For this review, take the finished solid that the model builds, in its own axes (mm). Face numbers are marked on the shaded views. A direction names the side the tool comes from. Coordinates: 2 decimals unless noted, no trailing zeros. Write each loop counter-clockwise with the first axis right and the second up, starting at its lowest first coordinate (ties: lowest second). Pieces come first, ordered by that corner, then holes.
1) We need section D-D on z = -5. Write out the cut boundary in (x, y), then the cut area to 3 significant figures.
2) We need section A-A on x = 0. Write out the cut boundary in (y, z), then the cut area to 4 significant figures.
3) We need section B-B on z = 73.5. Give the number of separate pieces and of enclosed holes in the cut face, then the cut area to 3 significant figures.
4) For the marked faces 5, 6 and 7, list the 3-axis set-ups (+Z, -Z, +X, -X, +Y, -Y) from which the entire face can be reached by the end or side of a thin tool; tool diameter is ignored.
5) To check wall thickness, follow line 1 along Z through (x, y) = (0, 0.5); line 2 along X through (y, z) = (9.25, 73.5); line 3 along X through (y, z) = (7, 21.5). State the ranges of each line that lie inside material, in increasing order.
6) We need section C-C on x = 5.5. Write out the cut boundary in (y, z), then the cut area to 4 significant figures.
7) Insertion check: P1, Ø1.5, axis at x = -19.5, z = 22, coming from the +Y side; P2, Ø12, axis at x = 5, z = 68, coming from the +Y side; P3, Ø1.9, axis at x = 17.5, z = 65, coming from the +Y side; P4, Ø2.5, axis at x = -17, z = 29.5, coming from the -Y side. Each pin has a flat end and moves straight along its axis. Give the tip position at first contact, or say it passes through.
8) Mouldability with a two-part tool opening along X and no side actions: class the marked faces 1, 2, 3 and 4 as pulls with the +X half, pulls with the -X half, needs draft (parallel to the pull), parting line crosses it, or undercut.
from build123d import *

# Parameters (mm, degrees)
BOSS_EXTRUDE1_DEPTH = 95
CUT_EXTRUDE1_DEPTH  = 1
CUT_EXTRUDE2_DEPTH  = 1
CUT_EXTRUDE4_DEPTH  = 2
CUT_EXTRUDE5_DEPTH  = 2
FILLET1_R           = 2
FILLET2_R           = 5
FILLET3_R           = 5
SKETCH11_R          = 3.25
SKETCH11_R_2        = 1.9
BOSS_EXTRUDE2_DEPTH = 1.5
SKETCH13_R          = 2.5
BOSS_EXTRUDE3_DEPTH = 7.4
SKETCH14_R          = 1.9
BOSS_EXTRUDE4_DEPTH = 1
SKETCH15_R          = 1.65
CUT_EXTRUDE7_DEPTH  = 15
SKETCH16_R          = 2.75
CUT_EXTRUDE8_DEPTH  = 1
SKETCH17_R          = 1
CUT_EXTRUDE9_DEPTH  = 2
SKETCH18_W          = 37.144162516
SKETCH18_H          = 8.058946384
CUT_EXTRUDE10_DEPTH = 3
SKETCH19_R          = 1
SKETCH19_R_2        = 1.4
CUT_EXTRUDE11_DEPTH = 3
SKETCH20_W          = 42.739965368
SKETCH20_H          = 1.5
BOSS_EXTRUDE5_DEPTH = 10
FILLET4_R           = 10
SKETCH21_W          = 42.739965368
SKETCH21_H          = 1.5
BOSS_EXTRUDE6_DEPTH = 10
FILLET5_R           = 10
SKETCH22_R          = 2.5
CUT_EXTRUDE12_DEPTH = 10
SKETCH23_R          = 2.5
CUT_EXTRUDE13_DEPTH = 4.5


with BuildPart() as part:
    # Sketch1 → Boss-Extrude1 (new body)
    with BuildSketch(Plane.XY):
        Polygon((-26.114805518, 0), (-27.425, 25), (-24.921569135, 25), (-23.742394101, 2.5), (23.742394101, 2.5), (24.921569135, 25), (27.425, 25), (26.114805518, 0), align=None)
    extrude(amount=BOSS_EXTRUDE1_DEPTH)

    # Sketch2 → Cut-Extrude1 (cut)
    with BuildSketch(Plane(origin=(23.546701863, -1.234030354, 0), x_dir=(0, 0, 1), z_dir=(-0.9986295347545742, 0.052335956242940705, 0))):
        Polygon((93, 3.739154736), (93, 24.853460661), (2, 24.853460661), (2, 3.739154736), (0, 3.739154736), (0, 26.853460661), (95, 26.853460661), (95, 3.739154736), align=None)
    extrude(amount=-CUT_EXTRUDE1_DEPTH, mode=Mode.SUBTRACT)

    # Sketch4 → Cut-Extrude2 (cut)
    with BuildSketch(Plane(origin=(-23.546701863, -1.234030354, 0), x_dir=(0, 0, -1), z_dir=(0.9986295347545742, 0.052335956242940414, 0))):
        Polygon((-95, 3.739154736), (-93, 3.739154736), (-93, 24.754638821), (-2, 24.754638821), (-2, 3.739154736), (0, 3.739154736), (0, 26.754638821), (-95, 26.754638821), align=None)
    extrude(amount=-CUT_EXTRUDE2_DEPTH, mode=Mode.SUBTRACT)

    # Sketch9 → Cut-Extrude4 (cut)
    with BuildSketch(Plane.XY.offset(95)):
        Polygon((-24.741023636, 2.447664044), (-24.691358668, 1.5), (24.691358668, 1.5), (24.743766447, 2.5), (23.742394101, 2.5), (-23.742394101, 2.5), (-24.743766447, 2.5), align=None)
    extrude(amount=-CUT_EXTRUDE4_DEPTH, mode=Mode.SUBTRACT)

    # Sketch10 → Cut-Extrude5 (cut)
    with BuildSketch(Plane(origin=(0, 0, 0), x_dir=(-1, 0, 0), z_dir=(0, 0, -1))):
        Polygon((-24.741023636, 2.447664044), (-24.691358668, 1.5), (24.691358668, 1.5), (24.741023636, 2.447664044), (24.743766447, 2.5), (23.742394101, 2.5), (-23.742394101, 2.5), (-24.743766447, 2.5), align=None)
    extrude(amount=-CUT_EXTRUDE5_DEPTH, mode=Mode.SUBTRACT)

    # Fillet1
    fillet1_edges = [part.edges().sort_by_distance(p)[0] for p in [
        (24.691358668, 1.5, 1),
        (-24.691358668, 1.5, 1),
        (23.742394101, 2.5, 47.5),
        (-23.742394101, 2.5, 47.5),
        (-24.691358668, 1.5, 94),
        (24.691358668, 1.5, 94),
    ]]
    fillet(fillet1_edges, radius=FILLET1_R)

    # Fillet2
    fillet2_edges = [part.edges().sort_by_distance(p)[0] for p in [
        (26.673970741, 25, 95),
        (25.34674626, 23.559201525, 93),
        (25.34674626, 23.559201525, 2),
        (-26.673970741, 25, 0),
        (-26.673970741, 25, 95),
        (-25.341574324, 23.460515117, 2),
        (-25.341574324, 23.460515117, 93),
        (26.673970741, 25, 0),
    ]]
    fillet(fillet2_edges, radius=FILLET2_R)

    # Fillet3
    fillet3_edges = [part.edges().sort_by_distance(p)[0] for p in [
        (-26.114805518, 0, 47.5),
        (26.114805518, 0, 47.5),
    ]]
    fillet(fillet3_edges, radius=FILLET3_R)

    # Sketch11 → Boss-Extrude2 (add)
    with BuildSketch(Plane(origin=(0, 2.5, 0), x_dir=(1, 0, 0), z_dir=(0, 1, 0))):
        with Locations(Location((-18.5, -21.5, 0), (0, 0, 90))):
            Circle(SKETCH11_R)
        with Locations(Location((18.5, -21.5, 0), (0, 0, 90))):
            Circle(SKETCH11_R)
        with Locations(Location((-17, -29.5, 0), (0, 0, 90))):
            Circle(SKETCH11_R_2)
        with Locations(Location((17, -29.5, 0), (0, 0, 90))):
            Circle(SKETCH11_R_2)
        with Locations(Location((18.5, -73.5, 0), (0, 0, 90))):
            Circle(SKETCH11_R)
        with Locations(Location((17, -65.5, 0), (0, 0, 90))):
            Circle(SKETCH11_R_2)
        with Locations(Location((-18.5, -73.5, 0), (0, 0, 90))):
            Circle(SKETCH11_R)
        with Locations(Location((-17, -65.5, 0), (0, 0, 90))):
            Circle(SKETCH11_R_2)
    extrude(amount=BOSS_EXTRUDE2_DEPTH)

    # Sketch13 → Boss-Extrude3 (add)
    with BuildSketch(Plane(origin=(0, 4, 0), x_dir=(1, 0, 0), z_dir=(0, 1, 0))):
        with Locations(Location((-18.5, -21.5, 0), (0, 0, 270))):
            Circle(SKETCH13_R)
        with Locations(Location((18.5, -21.5, 0), (0, 0, 270))):
            Circle(SKETCH13_R)
        with Locations(Location((-18.5, -73.5, 0), (0, 0, 90))):
            Circle(SKETCH13_R)
        with Locations(Location((18.5, -73.5, 0), (0, 0, 90))):
            Circle(SKETCH13_R)
    extrude(amount=BOSS_EXTRUDE3_DEPTH)

    # Sketch14 → Boss-Extrude4 (add)
    with BuildSketch(Plane(origin=(0, 4, 0), x_dir=(1, 0, 0), z_dir=(0, 1, 0))):
        with Locations(Location((-17, -29.5, 0), (0, 0, 90))):
            Circle(SKETCH14_R)
        with Locations(Location((17, -29.5, 0), (0, 0, 90))):
            Circle(SKETCH14_R)
        with Locations(Location((-17, -65.5, 0), (0, 0, 90))):
            Circle(SKETCH14_R)
        with Locations(Location((17, -65.5, 0), (0, 0, 90))):
            Circle(SKETCH14_R)
    extrude(amount=BOSS_EXTRUDE4_DEPTH)

    # Sketch15 → Cut-Extrude7 (cut)
    with BuildSketch(Plane(origin=(0, 11.4, 0), x_dir=(1, 0, 0), z_dir=(0, 1, 0))):
        with Locations(Location((-18.5, -21.5, 0), (0, 0, 270))):
            Circle(SKETCH15_R)
        with Locations(Location((18.5, -21.5, 0), (0, 0, 270))):
            Circle(SKETCH15_R)
        with Locations(Location((18.5, -73.5, 0), (0, 0, 270))):
            Circle(SKETCH15_R)
        with Locations(Location((-18.5, -73.5, 0), (0, 0, 270))):
            Circle(SKETCH15_R)
    extrude(amount=-CUT_EXTRUDE7_DEPTH, mode=Mode.SUBTRACT)

    # Sketch16 → Cut-Extrude8 (cut)
    with BuildSketch(Plane.XZ):
        with Locations((18.5, 21.5)):
            Circle(SKETCH16_R)
        with Locations((-18.5, 21.5)):
            Circle(SKETCH16_R)
        with Locations((18.5, 73.5)):
            Circle(SKETCH16_R)
        with Locations((-18.5, 73.5)):
            Circle(SKETCH16_R)
    extrude(amount=-CUT_EXTRUDE8_DEPTH, mode=Mode.SUBTRACT)

    # Sketch17 → Cut-Extrude9 (cut)
    with BuildSketch(Plane(origin=(0, 5, 0), x_dir=(1, 0, 0), z_dir=(0, 1, 0))):
        with Locations(Location((-17, -29.5, 0), (0, 0, 270))):
            Circle(SKETCH17_R)
        with Locations(Location((-17, -65.5, 0), (0, 0, 270))):
            Circle(SKETCH17_R)
        with Locations(Location((17, -65.5, 0), (0, 0, 270))):
            Circle(SKETCH17_R)
        with Locations(Location((17, -29.5, 0), (0, 0, 270))):
            Circle(SKETCH17_R)
    extrude(amount=-CUT_EXTRUDE9_DEPTH, mode=Mode.SUBTRACT)

    # Sketch18 → Cut-Extrude10 (cut)
    with BuildSketch(Plane(origin=(26.043275699, -1.364870245, 0), x_dir=(0, 0, -1), z_dir=(0.9986295347545742, -0.05233595624294077, 0))):
        with Locations((-47.623813875, 11.404221833)):
            Rectangle(SKETCH18_W, SKETCH18_H)
    extrude(amount=-CUT_EXTRUDE10_DEPTH, mode=Mode.SUBTRACT)

    # Sketch19 → Cut-Extrude11 (cut)
    with BuildSketch(Plane(origin=(-26.043275699, -1.364870245, 0), x_dir=(0, 0, 1), z_dir=(-0.9986295347545742, -0.05233595624294044, 0))):
        with Locations(Location((14.034522451, 8.411566152, 0), (0, 0, 270))):
            Circle(SKETCH19_R)
        with Locations(Location((34.99921548, 8.411566152, 0), (0, 0, 270))):
            Circle(SKETCH19_R)
        with Locations(Location((40.74921548, 11.111566152, 0), (0, 0, 270))):
            Circle(SKETCH19_R_2)
        with Locations(Location((45.99921548, 11.111566152, 0), (0, 0, 270))):
            Circle(SKETCH19_R_2)
        with Locations(Location((51.19921548, 11.111566152, 0), (0, 0, 270))):
            Circle(SKETCH19_R_2)
    extrude(amount=-CUT_EXTRUDE11_DEPTH, mode=Mode.SUBTRACT)

    # Sketch20 → Boss-Extrude5 (add)
    with BuildSketch(Plane(origin=(0, 0, 0), x_dir=(-1, 0, 0), z_dir=(0, 0, -1))):
        with Locations((0, 0.75)):
            Rectangle(SKETCH20_W, SKETCH20_H)
    extrude(amount=BOSS_EXTRUDE5_DEPTH)

    # Fillet4
    fillet4_edges = [part.edges().sort_by_distance(p)[0] for p in [
        (21.369982684, 0.75, -10),
        (-21.369982684, 0.75, -10),
    ]]
    fillet(fillet4_edges, radius=FILLET4_R - 0.0001)  # a hair under: the kernel refuses the full size

    # Sketch21 → Boss-Extrude6 (add)
    with BuildSketch(Plane.XY.offset(95)):
        with Locations((0, 0.75)):
            Rectangle(SKETCH21_W, SKETCH21_H)
    extrude(amount=BOSS_EXTRUDE6_DEPTH)

    # Fillet5
    fillet5_edges = [part.edges().sort_by_distance(p)[0] for p in [
        (-21.369982684, 0.75, 105),
        (21.369982684, 0.75, 105),
    ]]
    fillet(fillet5_edges, radius=FILLET5_R - 0.0001)  # a hair under: the kernel refuses the full size

    # Sketch22 → Cut-Extrude12 (cut)
    with BuildSketch(Plane(origin=(0, 1.5, 0), x_dir=(1, 0, 0), z_dir=(0, 1, 0))):
        with Locations(Location((0, 5, 0), (0, 0, 180))):
            Circle(SKETCH22_R)
        with Locations(Location((0, -100, 0), (0, 0, 180))):
            Circle(SKETCH22_R)
    extrude(amount=-CUT_EXTRUDE12_DEPTH, mode=Mode.SUBTRACT)

    # Sketch23 → Cut-Extrude13 (cut)
    with BuildSketch(Plane(origin=(-26.043275699, -1.364870245, 0), x_dir=(0, 0, 1), z_dir=(-0.9986295347545742, -0.052335956242940324, 0))):
        with Locations(Location((9.104177009, 17.111566152, 0), (0, 0, 270))):
            Circle(SKETCH23_R)
    extrude(amount=-CUT_EXTRUDE13_DEPTH, mode=Mode.SUBTRACT)


solid = part.part
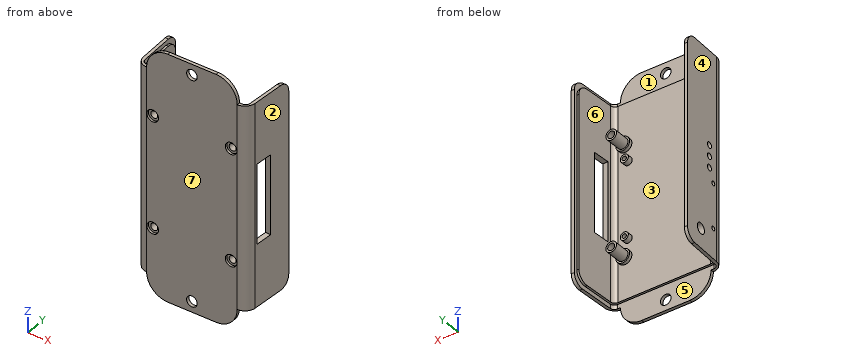
Result:
1. outline: (-20.03, 0) - (-2.5, 0) - (-2.5, 1.5) - (-20.03, 1.5) - close; (2.5, 0) - (20.03, 0) - (20.03, 1.5) - (2.5, 1.5) - close
1. area: 52.6 mm2
2. outline: (0, -10) - (1.5, -10) - (1.5, -7.5) - (0, -7.5) - close; (0, -2.5) - (1.5, -2.5) - (1.5, 2) - (2.5, 2) - (2.5, 93) - (1.5, 93) - (1.5, 97.5) - (0, 97.5) - close; (0, 102.5) - (1.5, 102.5) - (1.5, 105) - (0, 105) - close
2. area: 248.5 mm2
3. separate pieces: 3
3. enclosed holes: 0
3. area: 246 mm2
4. face 5: -Z, +Y
4. face 6: +Z, -Z, +Y
4. face 7: +Z, -Z, +X, -X, -Y
5. line 1: z = -10 to -7.5, -2.5 to 97.5, 102.5 to 105
5. line 2: x = -26.6 to -24.1, -21 to -20.15, -16.85 to -16, 16 to 16.85, 20.15 to 21, 24.1 to 26.6
5. line 3: x = -26.48 to -23.98, -21 to -20.15, -16.85 to -16, 16 to 16.85, 20.15 to 21, 23.98 to 26.48
6. outline: (0, -10) - (1.5, -10) - (1.5, 2) - (2.5, 2) - (2.5, 93) - (1.5, 93) - (1.5, 105) - (0, 105) - close
6. area: 263.5 mm2
7. P1: stops at y = 11.4
7. P2: stops at y = 2.5
7. P3: stops at y = 5
7. P4: stops at y = 0
8. face 1: undercut
8. face 2: pulls with the +X half
8. face 3: undercut
8. face 4: pulls with the -X half
